Part model, mm, in its own coordinate system. Coordinates: 2 decimals unless noted, no trailing zeros. Loops run counter-clockwise (first coordinate to the right, second up) from the corner with the lowest first, then second, coordinate; pieces in that order, holes last.
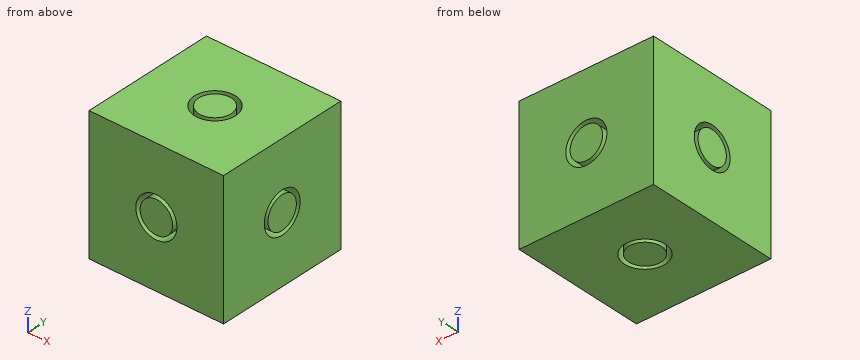
```python
from build123d import *

# Parameters (mm, degrees)
SKETCH1_W           = 55.3
SKETCH1_H           = 55.3
BOSS_EXTRUDE1_DEPTH = 27.65
SKETCH2_R           = 8.45
SKETCH2_R_2         = 6.7
CUT_EXTRUDE2_DEPTH  = 9.5
CUT_EXTRUDE3_START  = -9.5
SKETCH3_R           = 8.45
SKETCH3_R_2         = 6.7
CUT_EXTRUDE3_DEPTH  = 9.5
SKETCH4_R           = 8.45
SKETCH4_R_2         = 6.7
CUT_EXTRUDE4_DEPTH  = 9.5
CUT_EXTRUDE5_START  = -9.5
SKETCH5_R           = 8.45
SKETCH5_R_2         = 6.7
CUT_EXTRUDE5_DEPTH  = 9.5
SKETCH6_R           = 8.45
SKETCH6_R_2         = 6.7
CUT_EXTRUDE6_DEPTH  = 9.5
CUT_EXTRUDE7_START  = -9.5
SKETCH7_R           = 8.45
SKETCH7_R_2         = 6.7
CUT_EXTRUDE7_DEPTH  = 9.5


with BuildPart() as part:
    # Sketch1 → Boss-Extrude1 (new, symmetric)
    with BuildSketch(Plane(origin=(0, 0, 0), x_dir=(1, 0, 0), z_dir=(0, 1, 0))):
        Rectangle(SKETCH1_W, SKETCH1_H)
    extrude(amount=BOSS_EXTRUDE1_DEPTH, both=True)

    # Sketch2 → Cut-Extrude2 (cut)
    with BuildSketch(Plane(origin=(0, 27.65, 0), x_dir=(1, 0, 0), z_dir=(0, 1, 0))):
        with Locations(Location((0, 0, 0), (0, 0, 270))):
            Circle(SKETCH2_R)
        with Locations(Location((0, 0, 0), (0, 0, 270))):
            Circle(SKETCH2_R_2, mode=Mode.SUBTRACT)
    extrude(amount=-CUT_EXTRUDE2_DEPTH, mode=Mode.SUBTRACT)

    # Sketch3 → Cut-Extrude3 (cut)
    with BuildSketch(Plane.XZ.offset(27.65).offset(CUT_EXTRUDE3_START)):
        with Locations(Location((0, 0, 0), (0, 0, 90))):
            Circle(SKETCH3_R)
        with Locations(Location((0, 0, 0), (0, 0, 90))):
            Circle(SKETCH3_R_2, mode=Mode.SUBTRACT)
    extrude(amount=CUT_EXTRUDE3_DEPTH, mode=Mode.SUBTRACT)

    # Sketch4 → Cut-Extrude4 (cut)
    with BuildSketch(Plane(origin=(27.65, 0, 0), x_dir=(0, 0, -1), z_dir=(1, 0, 0))):
        Circle(SKETCH4_R)
        Circle(SKETCH4_R_2, mode=Mode.SUBTRACT)
    extrude(amount=-CUT_EXTRUDE4_DEPTH, mode=Mode.SUBTRACT)

    # Sketch5 → Cut-Extrude5 (cut)
    with BuildSketch(Plane.ZY.offset(27.65).offset(CUT_EXTRUDE5_START)):
        with Locations(Location((0, 0, 0), (0, 0, 180))):
            Circle(SKETCH5_R)
        with Locations(Location((0, 0, 0), (0, 0, 180))):
            Circle(SKETCH5_R_2, mode=Mode.SUBTRACT)
    extrude(amount=CUT_EXTRUDE5_DEPTH, mode=Mode.SUBTRACT)

    # Sketch6 → Cut-Extrude6 (cut)
    with BuildSketch(Plane.XY.offset(27.65)):
        Circle(SKETCH6_R)
        Circle(SKETCH6_R_2, mode=Mode.SUBTRACT)
    extrude(amount=-CUT_EXTRUDE6_DEPTH, mode=Mode.SUBTRACT)

    # Sketch7 → Cut-Extrude7 (cut)
    with BuildSketch(Plane(origin=(0, 0, -27.65), x_dir=(-1, 0, 0), z_dir=(0, 0, -1)).offset(CUT_EXTRUDE7_START)):
        with Locations(Location((0, 0, 0), (0, 0, 180))):
            Circle(SKETCH7_R)
        with Locations(Location((0, 0, 0), (0, 0, 180))):
            Circle(SKETCH7_R_2, mode=Mode.SUBTRACT)
    extrude(amount=CUT_EXTRUDE7_DEPTH, mode=Mode.SUBTRACT)


solid = part.part
```
Q1. Probe line 1 (X direction, y = 25, z = 0); line 2 (X direction, y = -20, z = 1). List the from-to ranges inside material, lowest first.
Q2. Saw through at A-A (y = -19). List the corners of the cut face in (x, z).
Q3. Saw through at C-C (x = 7.5). List the corners of the cut face in (y, z), plus the area to 3 significant figures.
Checked values:
1. line 1: x = -27.65 to -8.45, -6.7 to 6.7, 8.45 to 27.65
1. line 2: x = -27.65 to -8.39, -6.62 to 6.62, 8.39 to 27.65
2. outline: (-27.65, -27.65) - (27.65, -27.65) - (27.65, 27.65) - (-27.65, 27.65) - close; circle Ø13.4 at (0, 0); hole circle Ø16.9 at (0, 0)
3. outline: (-27.65, -27.65) - (-3.89, -27.65) - (-3.89, -18.15) - (3.89, -18.15) - (3.89, -27.65) - (27.65, -27.65) - (27.65, -3.89) - (18.15, -3.89) - (18.15, 3.89) - (27.65, 3.89) - (27.65, 27.65) - (3.89, 27.65) - (3.89, 18.15) - (-3.89, 18.15) - (-3.89, 27.65) - (-27.65, 27.65) - (-27.65, 3.89) - (-18.15, 3.89) - (-18.15, -3.89) - (-27.65, -3.89) - close
3. area: 2,760 mm2
